Source: CAD feature listing. Evaluate the final solid. Frame: model axes, mm. Face numbers are marked on the shaded views. A direction names the side the tool comes from. Round coordinates to 2 decimals unless told otherwise and drop trailing zeros. Order: outer loops, then holes, each group sorted by start corner. A loop starts at its lowest first (then second) coordinate and runs counter-clockwise, first axis right, second up. Notation, with made-up numbers: (53, -13.5) -> (72, -13.5) arc R24 cw to (72, -0.5) -> close; hole circle Ø8 at (74, 84.5). An arc over 180 degrees is marked (long way). Use a Markdown table: item, result. Add a question column.
```python
from build123d import *

# Parameters (mm, degrees)
EXTRUDE_THIN1_DEPTH     = 123.98756
CUT_EXTRUDE1_DEPTH      = 1
CUT_EXTRUDE1_DEPTH_BACK = 39.1
CUT_EXTRUDE2_DEPTH      = 1
CUT_EXTRUDE2_DEPTH_BACK = 39.1


with BuildPart() as part:
    # Sketch1 → Extrude-Thin1 (new body, symmetric)
    with BuildSketch(Plane(origin=(0, 0, 0), x_dir=(0, 0, -1), z_dir=(1, 0, 0))):
        with BuildLine():
            Line((-15.875, 19.05), (15.875, 19.05))
            ThreePointArc((15.875, 19.05), (18.12006403, 18.12006403), (19.05, 15.875))
            Line((19.05, 15.875), (19.05, -15.875))
            ThreePointArc((19.05, -15.875), (18.12006403, -18.12006403), (15.875, -19.05))
            Line((15.875, -19.05), (-15.875, -19.05))
            ThreePointArc((-15.875, -19.05), (-18.12006403, -18.12006403), (-19.05, -15.875))
            Line((-19.05, -15.875), (-19.05, 15.875))
            ThreePointArc((-19.05, 15.875), (-18.12006403, 18.12006403), (-15.875, 19.05))
        make_face()
        with BuildLine():
            Line((-15.875, 16.51), (15.875, 16.51))
            ThreePointArc((15.875, 16.51), (16.324012806, 16.324012806), (16.51, 15.875))
            Line((16.51, 15.875), (16.51, -15.875))
            ThreePointArc((16.51, -15.875), (16.324012806, -16.324012806), (15.875, -16.51))
            Line((15.875, -16.51), (-15.875, -16.51))
            ThreePointArc((-15.875, -16.51), (-16.324012806, -16.324012806), (-16.51, -15.875))
            Line((-16.51, -15.875), (-16.51, 15.875))
            ThreePointArc((-16.51, 15.875), (-16.324012806, 16.324012806), (-15.875, 16.51))
        make_face(mode=Mode.SUBTRACT)
    extrude(amount=EXTRUDE_THIN1_DEPTH, both=True)

    # Sketch3 → Cut-Extrude1 (cut, two sides)
    with BuildSketch(Plane(origin=(0, 19.05, 0), x_dir=(1, 0, 0), z_dir=(0, 1, 0))) as cut_extrude1_sk:
        Polygon((299.02319091, -499.956443526), (123.98756, -19.05), (110.120294074, 19.05), (-64.915336836, 499.956443526), (896.897550216, 850.027705346), (1260.836077962, -149.885181705), align=None)
    extrude(amount=CUT_EXTRUDE1_DEPTH, mode=Mode.SUBTRACT)
    extrude(cut_extrude1_sk.sketch, amount=-CUT_EXTRUDE1_DEPTH_BACK, mode=Mode.SUBTRACT)

    # Sketch4 → Cut-Extrude2 (cut, two sides)
    with BuildSketch(Plane(origin=(0, 19.05, 0), x_dir=(1, 0, 0), z_dir=(0, 1, 0))) as cut_extrude2_sk:
        Polygon((-340.270885768, -482.871088899), (-123.98756, -19.05), (-106.221238224, 19.05), (110.062087543, 482.871088899), (-817.580090255, 915.437740434), (-1267.913063566, -50.304437364), align=None)
    extrude(amount=CUT_EXTRUDE2_DEPTH, mode=Mode.SUBTRACT)
    extrude(cut_extrude2_sk.sketch, amount=-CUT_EXTRUDE2_DEPTH_BACK, mode=Mode.SUBTRACT)


solid = part.part
```
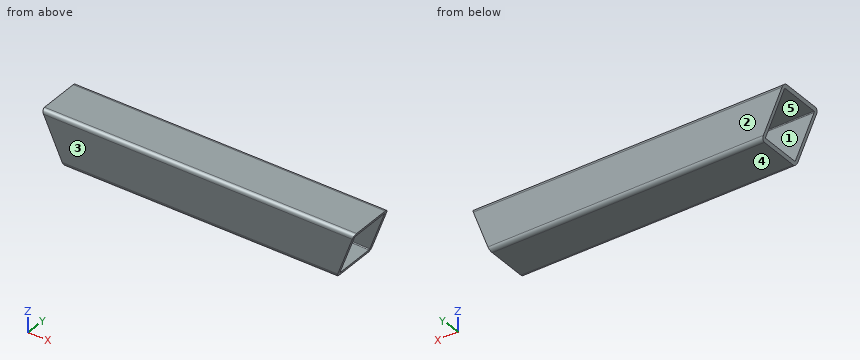
1) Section C-C on z = -1.5. Output: boundary loops of the cut face in (x, y).
2) First-contact query: pin 1 Ø12 at (y, z) = (4, 12.5) entering from -X; pin 2 Ø12 at (y, z) = (-10, -2.5) entering from +X. Flat tips, straight axial feed; report the tip coordinate or a pass-through.
3) Draft query along Y for the marked faces 3, 4 and 5. Return one class per face: pulls with the +Y half, pulls with the -Y half, needs draft (parallel to the pull), parting line crosses it, or undercut.
4) Reachability of the marked faces 1 and 2 from +Z, -Z, +X, -X, +Y, -Y: full face, straight path, thin tool, end or side. Return the list, or none.
5) Line query: probe 1 along Y at (x, z) = (96, -11.5); probe 2 along Z at (x, y) = (114.5, 16). Output: solid intervals per line, ascending. Write a range as from..to.
6) Section A-A on x = 23. Output: boundary loops of the cut face in (y, z) (3 decimals), then the cut area to 3 significant figures.
7) Section B-B on y = -4.5. Output: boundary loops of the cut face in (x, z).
Conclusion:
| question | item | result |
|---|---|---|
| 1 | outline | (-114.4, -19.05) -> (116.51, -19.05) -> (116.51, -16.51) -> (-114.4, -16.51) -> close; (-114.4, 16.51) -> (116.51, 16.51) -> (116.51, 19.05) -> (-114.4, 19.05) -> close |
| 2 | pin 1 | stops at x = -123.73 |
| 2 | pin 2 | passes through |
| 3 | face 3 | pulls with the -Y half |
| 3 | face 4 | needs draft |
| 3 | face 5 | undercut |
| 4 | face 1 | +X, -X |
| 4 | face 2 | +Z, -Z, +X, -X, +Y |
| 5 | probe 1 | y = -19.05..-16.51, 16.51..19.05 |
| 5 | probe 2 | z = 16.5..19.05 |
| 6 | outline | (-19.05, -15.875) arc R3.175 ccw to (-15.875, -19.05) -> (15.875, -19.05) arc R3.175 ccw to (19.05, -15.875) -> (19.05, 15.875) arc R3.175 ccw to (15.875, 19.05) -> (-15.875, 19.05) arc R3.175 ccw to (-19.05, 15.875) -> close; hole (-16.51, -15.875) arc R0.635 ccw to (-15.875, -16.51) -> (15.875, -16.51) arc R0.635 ccw to (16.51, -15.875) -> (16.51, 15.875) arc R0.635 ccw to (15.875, 16.51) -> (-15.875, 16.51) arc R0.635 ccw to (-16.51, 15.875) -> close |
| 6 | area | 353 mm^2 |
| 7 | outline | (-123.99, 19.05) -> (-122.8, 16.51) -> (123.06, 16.51) -> (123.99, 19.05) -> close; (-107.41, -16.51) -> (-106.22, -19.05) -> (110.12, -19.05) -> (111.04, -16.51) -> close |
